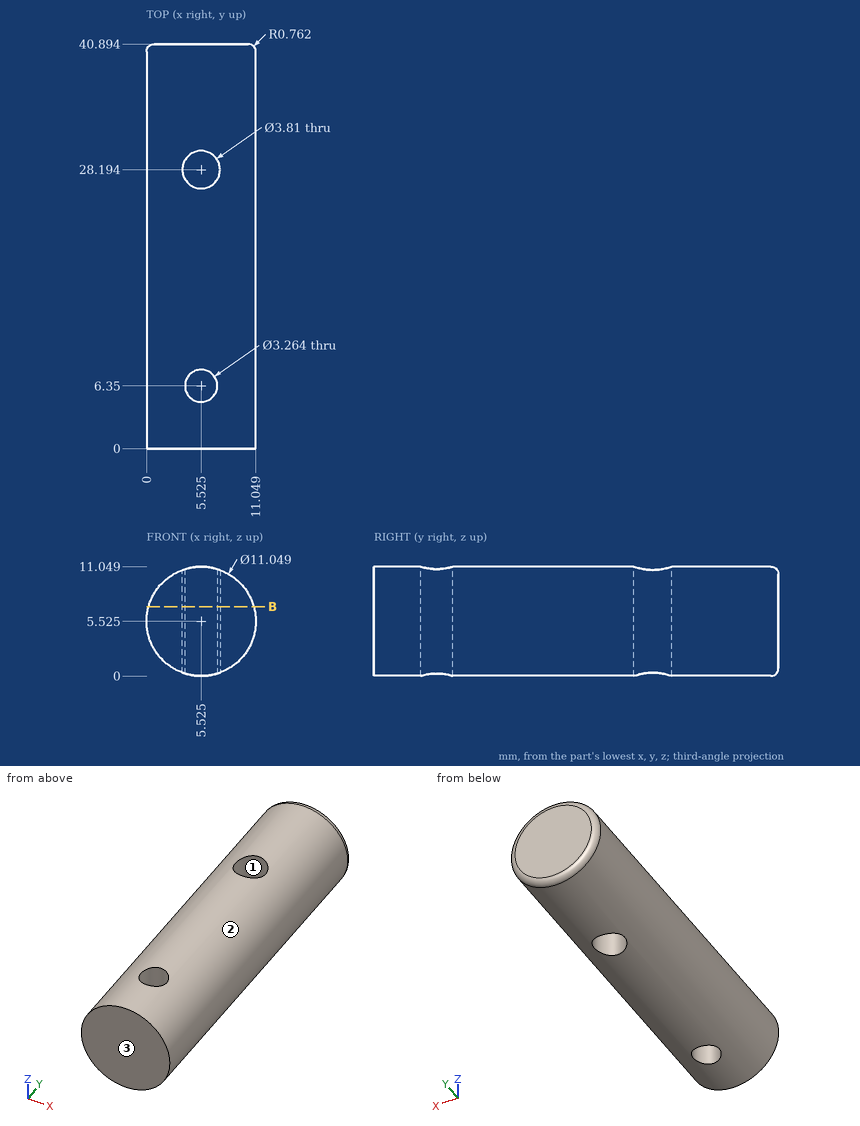
Could you check a few things on this drawing? It's one solid part, dimensions in mm from its lowest x, y, z. Give positions to 0.01 mm unless a question says otherwise; leave off trailing zeros. One line per item, written item: value. Start each with the question number.
1. If I drill on probe 1 along Y at (x, z) = (5.5, 6.75) (1 decimal); probe 2 along Y at (x, z) = (7.25, 7) (1 decimal); probe 3 along X at (y, z) = (18, 9.5), over which ranges is the centre line in solid material (lowest first)?
2. Imagine slicing it at B-B on z = 7. Give the number of separate pieces and of enclosed holes in the cut face.
3. Thinking about a two-plate mould opening in X: for the marked faces 1, 2 and 3, which applies, +X half, -X half, draft (parallel to the pull), parting line (faces both ways), or undercut?
4. For P1, Ø1, axis at x = 9, y = 6, coming from the +Z side; P2, Ø2, axis at x = 2, y = 19.5, coming from the -Z side; P3, Ø1, axis at x = 4, y = 14.5, coming from the +Z side, each with a flat end and sliding along its axis, tell me the tip position at first contact or that it passes through.
Values:
1. probe 1: 0 to 4.7, 8 to 26.3, 30.1 to 40.9
1. probe 2: 0 to 27.4, 29 to 40.9
1. probe 3: 1.69 to 9.36
2. separate pieces: 1
2. enclosed holes: 2
3. face 1: undercut
3. face 2: parting line
3. face 3: draft
4. P1: z = 10.18
4. P2: z = 0.61
4. P3: z = 10.95
